Here's how the part is built. I have some questions about the finished solid (model axes, mm). A direction names the side the tool comes from. Give positions to 0.01 mm unless a question says otherwise; leave off trailing zeros. Write each loop counter-clockwise with the first axis right and the second up, starting at its lowest first coordinate (ties: lowest second). Pieces come first, ordered by that corner, then holes. Notation, with made-up numbers: M 3.25,38.5 L 38.25,38.5 A17 ccw 38.25,71.5 Z; hole C -35.75,64 d9. An arc over 180 degrees is marked long. Answer as CSV lines item,"result". Start each with the question number.
Q1. Thinking about a two-plate mould opening in Y: for faces 1 (the flat face through (8, 13, 9)), 2 (the cylindrical face through (14.899, -1.504, 6.302)), 3 (the flat face through (-8.648, 13.028, 9.895)), which applies, +Y half, -Y half, draft (parallel to the pull), parting line (faces both ways), or undercut?
Q2. For pin 1 (4.5 mm diameter, centred on x = 2.5, z = 6.5, fed in from -Y); pin 2 (2.5 mm diameter, centred on x = 19.32, z = 17.5, fed in from -Y); pin 3 (0.9 mm diameter, centred on x = 12.5, y = 2.5, fed in from -Z), each with a flat end and sliding along its axis, tell me the tip position at first contact or that it passes through.
Q3. On a 3-axis mill with a long thin cutter (end or side, diameter ignored), from which of +Z, -Z, +X, -X, +Y, -Y can I reach the whole of each face in a straight line? I mean faces 4 (the flat face through (10, 6, 2.5)), 5 (the flat face through (19, -13, 17)), 6 (the cylindrical face through (14.48, 2.31, 5.7)). Say none if no direction works.
Q4. Suppose I cut it at C-C (y = -19.5). Write out the boundary of the cut face in (x, z).
Q5. Suppose I cut it at B-B (x = -1). Write out the boundary of the cut face in (y, z), then the cut area to 3 significant figures.
Q6. Suppose I cut it at A-A (z = 13.25). Write out the boundary of the cut face in (x, y), then the cut area to 3 significant figures.
Q7. If I drill on line 1 along Y through (x, z) = (14, 3.75); line 2 along X through (y, z) = (2.75, 5.25); line 3 along Y through (x, z) = (8.5, 4), over which ranges is the centre line in solid material (lowest first)?
Q8. Suppose I cut it at D-D (y = 7.5). Write out the boundary of the cut face in (x, z).
```python
from build123d import *

# Parameters (mm, degrees)
F0_R      = 5.5
F1_DEPTH  = 20
F2_R      = 5
F3_W      = 28
F3_H      = 10
F4_DEPTH  = 19
F5_W      = 14
F5_H      = 15
F6_DEPTH  = 2.5
F7_R      = 5
F8_R      = 5.05
F9_DEPTH  = 33
F10_R     = 1.65
F11_DEPTH = 9.5
F12_R     = 1.470884
F13_DEPTH = 6.5


with BuildPart() as f1:
    # F0 (on Top) → F1 (new body)
    with BuildSketch(Plane.XY):
        Polygon((22.324427, -26.5), (22.324427, 7), (14.324427, 15), (-6.675573, 15), (-10.675573, 11), (-10.675573, 4), (-6.675573, 0), (16.324427, 0), (16.324427, -26.5), align=None)
        with Locations((-3.675573, 7.5)):
            Circle(F0_R, mode=Mode.SUBTRACT)
    extrude(amount=F1_DEPTH)

    # F2
    f2_edges = [f1.edges().sort_by_distance(p)[0] for p in [
        (16.324427, 0, 10),
    ]]
    fillet(f2_edges, radius=F2_R)

    # F3 (on face) → F4 (cut)
    with BuildSketch(Plane.YZ.offset(22.324427)):
        with Locations((1, 15)):
            Rectangle(F3_W, F3_H)
    extrude(amount=-F4_DEPTH, mode=Mode.SUBTRACT)

    # F5 (on face) → F6 (cut)
    with BuildSketch(Plane.XY.offset(20)):
        with Locations((-3.675573, 7.5)):
            Rectangle(F5_W, F5_H)
    extrude(amount=-F6_DEPTH, mode=Mode.SUBTRACT)

    # F7
    f7_edges = [f1.edges().sort_by_distance(p)[0] for p in [
        (19.324427, -13, 10),
    ]]
    fillet(f7_edges, radius=F7_R)

    # F8 (on face) → F9 (cut)
    with BuildSketch(Plane.YZ.offset(22.324427)):
        with BuildLine():
            Line((-13, -2.5), (-13, -12.279106))
            Line((-13, -12.279106), (27.693347, -12.279106))
            Line((27.693347, -12.279106), (27.693347, 2.5))
            Line((27.693347, 2.5), (-8, 2.5))
            ThreePointArc((-8, 2.5), (-11.535534, 1.035534), (-13, -2.5))
        make_face()
        with Locations((-27.5, 10)):
            Circle(F8_R)
    extrude(amount=-F9_DEPTH, mode=Mode.SUBTRACT)

    # F10 (on face) → F11 (cut)
    with BuildSketch(Plane.XZ.offset(26.5)):
        with Locations((19.324427, 17.5)):
            Circle(F10_R)
        with Locations((19.324427, 2.5)):
            Circle(F10_R)
    extrude(amount=-F11_DEPTH, mode=Mode.SUBTRACT)

    # F12 (on face) → F13 (cut)
    with BuildSketch(Plane(origin=(0, 0, 2.5), x_dir=(1, 0, 0), z_dir=(0, 0, -1))):
        with Locations((7.574427, -2.75)):
            Circle(F12_R)
        with Locations((7.574427, -13.25)):
            Circle(F12_R)
        with Locations((13.074427, -2.75)):
            Circle(F12_R)
        with Locations((13.074427, -13.25)):
            Circle(F12_R)
    extrude(amount=-F13_DEPTH, mode=Mode.SUBTRACT)


solid = f1.part
```
Resolved:
1,face 1,"undercut"
1,face 2,"-Y half"
1,face 3,"+Y half"
2,pin 1,"y = 0"
2,pin 2,"y = -17"
2,pin 3,"z = 9"
3,face 4,"-Z, +X, -X, +Y"
3,face 5,"+Z, +X, -X, +Y"
3,face 6,"-Z"
4,outline,"M 16.32,0 L 22.32,0 L 22.32,20 L 16.32,20 Z; hole C 19.32,2.5 d3.3; hole C 19.32,17.5 d3.3"
5,outline,"M 0,2.5 L 2.69,2.5 L 2.69,17.5 L 0,17.5 Z; M 12.31,2.5 L 15,2.5 L 15,17.5 L 12.31,17.5 Z"
5,area,"80.8 mm^2"
6,outline,"M -10.68,4 L -6.68,0 L 3.32,0 L 3.32,15 L -6.68,15 L -10.68,11 Z; M 16.32,-23.63 L 22.32,-23.63 L 22.32,-12.68 L 16.32,-12.68 Z; hole C -3.68,7.5 d11"
6,area,"165 mm^2"
7,line 1,"-0.78 to 1.61, 3.89 to 12.11, 14.39 to 15"
7,line 2,"-9.43 to -6.45, -0.9 to 6.1, 9.05 to 11.6, 14.55 to 22.32"
7,line 3,"0 to 1.61, 3.89 to 12.11, 14.39 to 15"
8,outline,"M -10.68,2.5 L -9.18,2.5 L -9.18,17.5 L -10.68,17.5 Z; M 1.82,2.5 L 21.82,2.5 L 21.82,10 L 3.32,10 L 3.32,17.5 L 1.82,17.5 Z"
